Autodesk Inventor part; units mm, degrees
ref_plane "YZ Plane" through (0, 0, 0) normal (1, 0, 0) x (0, 1, 0)
ref_plane "XZ Plane" through (0, 0, 0) normal (0, 1, 0) x (-1, 0, 0)
ref_plane "XY Plane" through (0, 0, 0) normal (0, 0, 1) x (1, 0, 0)
sketch "Szkic1" plane through (0, 0, 0) normal (0, 1, 0) x (-1, 0, 0)
  line L0 (-50, 50) -> (50, 50)
  line L1 (50, 50) -> (50, -50)
  line L2 (50, -50) -> (-50, -50)
  line L3 (-50, -50) -> (-50, 50)
  line L4 (-50, 50) -> (50, -50) construction
  line L5 (50, 50) -> (-50, -50) construction
  point P0 (0, 0)
  dimension "d0" = 100
  dimension "d1" = 100
extrude "Wyciągnięcie proste1" add sketch "Szkic1" along normal blind 5
sketch "Szkic2" plane through (0, 5, 0) normal (0, 1, 0) x (1, 0, 0)
  line L0 (10, 0) -> (-10, 0)
  line L1 (-10, 0) -> (-10, -5)
  line L2 (-10, -5) -> (10, -5)
  line L3 (10, -5) -> (10, 0)
  point P0 (0, 0)
  dimension "d4" = 20
  dimension "d5" = 10
  dimension "d6" = 5
  dimension "d7" = 0
extrude "Wyciągnięcie proste2" add sketch "Szkic2" along normal blind 30
fillet "Zaokrąglenie1" radius 10 1 edges at (10, 35, 2.5)
fillet "Zaokrąglenie2" radius 10 1 edges at (-10, 35, 2.5)
sketch "Szkic3" plane through (-10, 5, 5) normal (0, 0, 1) x (1, 0, 0)
  arc A0 (20, 20) -> (0, 20) centre (10, 20) ccw
  point P0 (10, -5)
hole "Otwór1" at (0, 25, 5) direction (0, 0, -1) diameter 3.2 end through all
properties part number "podstawa"
Input: part model. Units: mm. Frame: model coordinates. A direction names the side the tool comes from. Round coordinates to 2 decimals unless told otherwise and drop trailing zeros. Loops run counter-clockwise (first coordinate to the right, second up) from the corner with the lowest first, then second, coordinate; pieces in that order, holes last. Notation, with made-up numbers: (44.5, 59) -> (52.5, 59) arc R24 ccw to (52.5, 76) -> close; hole circle Ø7 at (-2.5, -13). An arc over 180 degrees is marked (long way). Use one line per item in the form item = value. Start each with the question number.
Item 1: Contact query for flat-ended pins moving along their axis: pin 1 Ø4 at (y, z) = (13.5, 3) entering from -X; pin 2 Ø16 at (x, y) = (-4, 17.5) entering from +Z; pin 3 Ø10 at (y, z) = (24, 14) entering from -X; pin 4 Ø5.5 at (y, z) = (17, 3) entering from +X. Output: stop coordinate, or through.
Item 2: Mould query, pull axis Y, two halves, no side actions, for faces 6 (the face through (-1, 2, -50)), 7 (the face through (6.99, 32.15, 2.46)), 8 (the face through (-1.08, 26.18, 2.46)). Classes: pulls with the +Y half, pulls with the -Y half, needs draft (parallel to the pull), parting line crosses it, or undercut.
Item 3: Section query C-C on y = 11.5. Return the cut outline in (x, z).
Item 4: Set-up query: faces 1 (the face through (-50, 2, 1)), 2 (the face through (-10, 15, 2)), 3 (the face through (0, 20, 5)), 4 (the face through (10, 15, 3)), 5 (the face through (0, 20, 0)). Return all of +Z, -Z, +X, -X, +Y, -Y with unobstructed straight access to the full face (end or side cutting, diameter ignored); none if empty.
Item 5: Section query B-B on z = -22. Return the cut outline in (x, y), then the cut area to 3 significant figures.
Item 6: Material intervals for L1, parallel to Y at x = 0, z = 2; L2, parallel to Y at x = -17, z = 45.5, sorted ascending. Write a range as from..to.
Item 7: Section query A-A on x = 3.5. Return the cut outline in (y, z).
Ans:
q1.pin_1 = -10
q1.pin_2 = 5
q1.pin_3 = through
q1.pin_4 = 10
q2.face_6 = needs draft
q2.face_7 = pulls with the +Y half
q2.face_8 = undercut
q3.outline = (-10, 0) -> (10, 0) -> (10, 5) -> (-10, 5) -> close
q4.face_1 = +Z, -Z, -X, +Y, -Y
q4.face_2 = +Z, -Z, -X, +Y
q4.face_3 = +Z, +X, -X, +Y
q4.face_4 = +Z, -Z, +X, +Y
q4.face_5 = -Z, +X, -X, +Y
q5.outline = (-50, 0) -> (50, 0) -> (50, 5) -> (-50, 5) -> close
q5.area = 500 mm^2
q6.L1 = 0..23.4, 26.6..35
q6.L2 = 0..5
q7.outline = (0, -50) -> (5, -50) -> (5, 0) -> (34.37, 0) -> (34.37, 5) -> (5, 5) -> (5, 50) -> (0, 50) -> close
